The figure shows three views and two pictorial views of one solid part (mm, origin at its lowest corner). Answer the questions. A direction names the side the tool comes from. Give positions to 0.01 mm unless a question says otherwise; leave off trailing zeros. Write each loop counter-clockwise with the first axis right and the second up, starting at its lowest first coordinate (ties: lowest second). Pieces come first, ordered by that corner, then holes. Notation, with made-up numbers: (-14.5, 78) -> (1.5, 78) arc R11 ccw to (1.5, 89) -> close; hole circle Ø2 at (45.25, 45). An arc over 180 degrees is marked (long way). Write item = value, one per line. Start each with the question number.
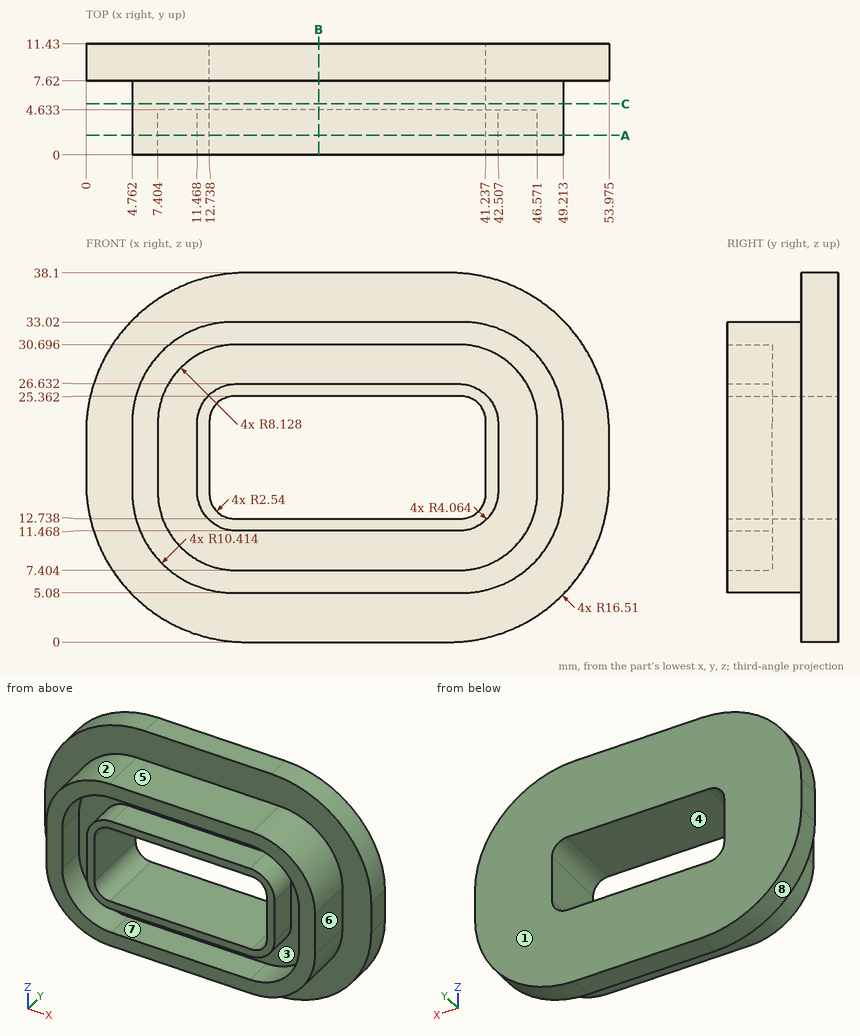
(1) A cutting plane is placed at C-C, the plane y = 5.25. Write down the section's boundary in (x, z) (1 decimal).
(2) A cutting plane is placed at B-B, the plane x = 24. Write down the section's boundary in (y, z) (1 decimal), then the cut area to 3 significant figures.
(3) A cutting plane is placed at A-A, the plane y = 2. State how many separate pieces and enclosed holes the cut face has.
(4) Each of these flat-tipped pins is pushed along its axis until it touches: pin 1 (2.5 mm diameter, centred on y = 1.5, z = 20.5, fed in from +X); pin 2 (3 mm diameter, centred on x = 12, y = 1.5, fed in from +Z); pin 3 (2.5 mm diameter, centred on x = 31.5, y = 2, fed in from +Z). Where does it stop, or does it pass through?
(5) Find the intervals of material crossed by line 1 along X through (y, z) = (3.25, 22) (1 decimal); line 2 along Z through (x, y) = (38, 3.5) (1 decimal); line 3 along Z through (x, y) = (20.5, 7.5), in increasing order.
(6) For the marked faces 1, 2, 3, 4 and 5, determine the directions among +Z, -Z, +X, -X, +Y, -Y from which every point of the face is accessible in a straight line to the end or side of a thin tool.
(7) Determine the mould class of the marked faces 6, 7 and 8 for opening direction Z: pulls with the +Z half, pulls with the -Z half, needs draft (parallel to the pull), parting line crosses it, or undercut.
Results list:
q1.outline = (4.8, 15.5) arc R10.4 ccw to (15.2, 5.1) -> (38.8, 5.1) arc R10.4 ccw to (49.2, 15.5) -> (49.2, 22.6) arc R10.4 ccw to (38.8, 33) -> (15.2, 33) arc R10.4 ccw to (4.8, 22.6) -> close; hole (12.7, 15.3) arc R2.5 ccw to (15.3, 12.7) -> (38.7, 12.7) arc R2.5 ccw to (41.2, 15.3) -> (41.2, 22.8) arc R2.5 ccw to (38.7, 25.4) -> (15.3, 25.4) arc R2.5 ccw to (12.7, 22.8) -> close
q2.outline = (0, 5.1) -> (7.6, 5.1) -> (7.6, 0) -> (11.4, 0) -> (11.4, 12.7) -> (0, 12.7) -> (0, 11.5) -> (4.6, 11.5) -> (4.6, 7.4) -> (0, 7.4) -> close; (0, 25.4) -> (11.4, 25.4) -> (11.4, 38.1) -> (7.6, 38.1) -> (7.6, 33) -> (0, 33) -> (0, 30.7) -> (4.6, 30.7) -> (4.6, 26.6) -> (0, 26.6) -> close
q2.area = 176 mm²
q3.separate_pieces = 2
q3.enclosed_holes = 2
q4.pin_1 = 49.21
q4.pin_2 = 32.88
q4.pin_3 = 33.02
q5.line_1 = 4.8 to 7.4, 11.5 to 12.7, 41.2 to 42.5, 46.6 to 49.2
q5.line_2 = 5.1 to 7.4, 11.5 to 12.7, 25.4 to 26.6, 30.7 to 33
q5.line_3 = 5.08 to 12.74, 25.36 to 33.02
q6.face_1 = +Z, -Z, +X, -X, +Y
q6.face_2 = +Z, -X, -Y
q6.face_3 = -Y
q6.face_4 = +Y, -Y
q6.face_5 = +Z, +X, -X, -Y
q7.face_6 = needs draft
q7.face_7 = undercut
q7.face_8 = pulls with the -Z half
